CAD build for the part. Positions are in the model's coordinates, mm. A direction names the side the tool comes from. Give positions to 0.01 mm unless a question says otherwise; leave off trailing zeros. Write each loop counter-clockwise with the first axis right and the second up, starting at its lowest first coordinate (ties: lowest second). Pieces come first, ordered by that corner, then holes. Notation, with made-up numbers: (54, -6) - (106, -6) arc R13 ccw to (106, 5) - close; hole circle Ø5 at (63, 53.25). An arc over 180 degrees is marked (long way). Answer as a JSON object with one key per item and string values.
from build123d import *

# Parameters (mm, degrees)
F0_W         = 150
F0_H         = 50
F1_DEPTH     = 100
F2_R         = 30
F3_DEPTH     = 40
F4_R         = 16
F5_R         = 16
F6_T1_DEPTH  = 75.1469278075
F6_T3_DEPTH  = 125.1469278075
F6_T5_DEPTH  = 175.1469278075
F6_T7_DEPTH  = 118
F6_T10_ANGLE = 90
F6_T12_ANGLE = 90
F6_T14_ANGLE = 90
F6_T18_DEPTH = 125.1469278075
F6_S19_R     = 30
F6_T20_DEPTH = 65
F7_R         = 6.3155551437
F8_DEPTH     = 2.4
F9_R         = 17.6407421848
F10_DEPTH    = 18


# Not quite as in the source:
# - a fillet or chamfer that OpenCascade refuses, or shapes differently, is made with other operations: its cross-section is extruded or revolved along the edge and cut away or added


with BuildPart() as f1:
    # F0 (on Top) → F1 (new body)
    with BuildSketch(Plane.XY):
        with Locations((-90.5639529228, -72.1464735391)):
            Rectangle(F0_W, F0_H)
    extrude(amount=F1_DEPTH)

    # F2 (on face) → F3 (join)
    with BuildSketch(Plane.XZ.offset(97.1464735391)):
        with Locations((-55.3404204547, 44.8933616281)):
            Circle(F2_R)
    extrude(amount=F3_DEPTH)

    # F4
    f4_edges = [f1.edges().sort_by_distance(p)[0] for p in [
        (-165.563953, -72.146474, 100),
    ]]
    fillet(f4_edges, radius=F4_R)

    # F5
    f5_edges = [f1.edges().sort_by_distance(p)[0] for p in [
        (-15.563953, -72.146474, 100),
        (-82.563953, -47.146474, 100),
    ]]
    fillet(f5_edges, radius=F5_R)

    # F6: chamfer of 16 on 4 edges, made by hand

    # F6_s2 → F6_t1 (cut)
    with BuildSketch(Plane.XZ.offset(63.1464735391)):
        Polygon((-149.5639529228, 0), (-165.5639529228, 16), (-165.5639529228, 0), align=None)
    extrude(amount=F6_T1_DEPTH, mode=Mode.SUBTRACT)

    # F6_s4 → F6_t3 (cut)
    with BuildSketch(Plane.XY.offset(-41.1469278075)):
        Polygon((-165.5639529228, -81.1464735391), (-149.5639529228, -97.1464735391), (-165.5639529228, -97.1464735391), align=None)
    extrude(amount=F6_T3_DEPTH, mode=Mode.SUBTRACT)

    # F6_s6 → F6_t5 (cut)
    with BuildSketch(Plane.YZ.offset(-149.5639529228)):
        Polygon((-47.1464735391, 16), (-63.1464735391, 0), (-47.1464735391, 0), align=None)
    extrude(amount=F6_T5_DEPTH, mode=Mode.SUBTRACT)

    # F6_s8 → F6_t7 (cut)
    with BuildSketch(Plane.YZ.offset(-149.5639529228)):
        Polygon((-97.1464735391, 84), (-81.1464735391, 100), (-97.1464735391, 100), align=None)
    extrude(amount=F6_T7_DEPTH, mode=Mode.SUBTRACT)

    # F6_s9 → F6_t10 (revolve, cut)
    with BuildSketch(Plane.YZ.offset(-149.5639529228)):
        Polygon((-63.1464735391, 0), (-47.1464735391, 16), (-47.1464735391, 0), align=None)
    revolve(axis=Axis((-149.5639529228, -63.1464735391, 0), (0, 0, 1)), revolution_arc=F6_T10_ANGLE, mode=Mode.SUBTRACT)

    # F6_s11 → F6_t12 (revolve, cut)
    with BuildSketch(Plane.XY.offset(84)):
        Polygon((-149.5639529228, -97.1464735391), (-165.5639529228, -81.1464735391), (-165.5639529228, -97.1464735391), align=None)
    revolve(axis=Axis((-149.5639529228, -97.1464735391, 84), (0, 1, 0)), revolution_arc=F6_T12_ANGLE, mode=Mode.SUBTRACT)

    # F6_s13 → F6_t14 (revolve, cut)
    with BuildSketch(Plane.YZ.offset(-31.5639529228)):
        Polygon((-97.1464735391, 84), (-81.1464735391, 100), (-97.1464735391, 100), align=None)
    revolve(axis=Axis((-31.5639529228, -97.1464735391, 84), (0, 1, 0)), revolution_arc=F6_T14_ANGLE, mode=Mode.SUBTRACT)


with BuildPart() as f6_tool16:
    # F6_s17 → F6_t18 (new body)
    with BuildSketch(Plane.XY.offset(-41.1469278075)):
        Polygon((-15.5639529228, -81.1464735391), (-31.5639529228, -97.1464735391), (-15.5639529228, -97.1464735391), align=None)
    extrude(amount=F6_T18_DEPTH)

    # F6_s19 → F6_t20 (cut, symmetric)
    with BuildSketch(Plane.XZ.offset(89.1)):
        with Locations((-55.3404204547, 44.8933616281)):
            Circle(F6_S19_R)
    extrude(amount=F6_T20_DEPTH, both=True, mode=Mode.SUBTRACT)


with BuildPart() as f1_1:
    add(f1.part)

    # F6_t15: cut F6_tool16
    add(f6_tool16.part, mode=Mode.SUBTRACT)

    # F7 (on face) → F8 (join)
    with BuildSketch(Plane.XY.offset(100)):
        with Locations((-52.6833832264, -69.3942382932)):
            Circle(F7_R)
    extrude(amount=F8_DEPTH)

    # F9 (on face) → F10 (join)
    with BuildSketch(Plane.XZ.offset(137.1464735391)):
        with Locations((-54.6616874635, 46.6945059597)):
            Circle(F9_R)
    extrude(amount=F10_DEPTH)


solid = f1_1.part
(1) Saw through at B-B, the plane z = 10. Give the cut face in (x, y), and give its area (3 significant figures).
Answer key:
{"outline": "(-159.56, -87.15) - (-149.56, -97.15) - (-31.56, -97.15) - (-15.56, -81.15) - (-15.56, -53.15) - (-149.56, -53.15) arc R10 ccw to (-159.56, -63.15) - close", "area": "6,140 mm²"}
(2) 3-axis set-ups, long thin cutter, end or side, ignore diameter. For faces 1 (the face through (-84, -80, 0)), 2 (the face through (-38.366, -146.02, 39.938)), 3 (the face through (-53.506, -63.132, 101.183)): which of +Z, -Z, +X, -X, +Y, -Y reach the whole face in a straight line?
Answer key:
{"face 1": "-Z, +X, -X, +Y, -Y", "face 2": "-Y", "face 3": "+Z"}
(3) Flat gauge pins, fed straight in: P1, Ø8, axis at y = -139, z = 19, coming from the +X side; P2, Ø9, axis at x = -76, y = -70, coming from the +Z side; P3, Ø4, axis at x = -82, z = 13.5, coming from the +Y side. Where does each tip first touch, or does it go through?
Answer key:
{"P1": "stops at x = -35.33", "P2": "stops at z = 100", "P3": "stops at y = -47.65"}
(4) Saw through at A-A, the plane x = -88. Give the cut face in (y, z).
Answer key:
{"outline": "(-97.15, 0) - (-63.15, 0) - (-47.15, 16) - (-47.15, 84) arc R16 ccw to (-63.15, 100) - (-81.15, 100) - (-97.15, 84) - close"}
(5) Probe L1, parallel to Y at x = -64, z = 30; L2, parallel to Y at x = -137.5, z = 37.5; L3, parallel to X at y = -140, z = 53.5. List the from-to ranges inside material, lowest first. Write a range as [from, to].
Answer key:
{"L1": "y = [-137.15, -47.15]", "L2": "y = [-97.15, -47.15]", "L3": "x = [-70.94, -38.39]"}
(6) Saw through at C-C, the plane y = -95. Give the cut face in (x, z).
Answer key:
{"outline": "(-151.71, 2.15) - (-149.56, 0) - (-29.42, 0) - (-29.42, 29.79) arc R30 ccw to (-29.42, 59.99) - (-29.42, 84) arc R2.15 ccw to (-31.56, 86.15) - (-149.56, 86.15) arc R2.15 ccw to (-151.71, 84) - close"}
(7) Saw through at D-D, the plane x = -56.5. Give the cut face in (y, z).
Answer key:
{"outline": "(-155.15, 29.15) - (-137.15, 29.15) - (-137.15, 14.92) - (-97.15, 14.92) - (-97.15, 0) - (-63.15, 0) - (-47.15, 16) - (-47.15, 84) arc R16 ccw to (-63.15, 100) - (-64.36, 100) - (-64.36, 102.4) - (-74.43, 102.4) - (-74.43, 100) - (-81.15, 100) - (-97.15, 84) - (-97.15, 74.87) - (-137.15, 74.87) - (-137.15, 64.24) - (-155.15, 64.24) - close"}
